from build123d import *

# Parameters (mm, degrees)
SKETCH_1_W      = 22.8
SKETCH_1_H      = 11.8
EXTRUDE_1_DEPTH = 22.6
SKETCH_2_R      = 5.9
EXTRUDE_2_DEPTH = 2.6
SKETCH_3_R      = 2.275
EXTRUDE_3_DEPTH = 2.6
EXTRUDE_4_DEPTH = 2.6
EXTRUDE_5_DEPTH = 2.5
SKETCH_6_W      = 1.6
SKETCH_6_H      = 4
EXTRUDE_6_DEPTH = 1.5
FILLET_1_R      = 0.4


with BuildPart() as part:
    # Эскиз1 → Бобышка-Вытянуть1 (new body)
    with BuildSketch(Plane.XY):
        Rectangle(SKETCH_1_W, SKETCH_1_H)
    extrude(amount=EXTRUDE_1_DEPTH)

    # Эскиз2 → Бобышка-Вытянуть2 (add)
    with BuildSketch(Plane.XY.offset(22.6)):
        with Locations((-5.5, 0)):
            Circle(SKETCH_2_R)
    extrude(amount=EXTRUDE_2_DEPTH)

    # Эскиз3 → Бобышка-Вытянуть3 (add)
    with BuildSketch(Plane.XY.offset(25.2)):
        with Locations((-5.5, 0)):
            Circle(SKETCH_3_R)
    extrude(amount=EXTRUDE_3_DEPTH)

    # Эскиз4 → Бобышка-Вытянуть4 (add)
    with BuildSketch(Plane.XY.offset(22.6)):
        with BuildLine():
            ThreePointArc((-0.419607843, 2.999935921), (-3.4, 0), (-0.419607843, -2.999935921))
            ThreePointArc((-0.419607843, -2.999935921), (0.4, 0), (-0.419607843, 2.999935921))
        make_face()
        with BuildLine():
            ThreePointArc((-0.419607843, 2.999935921), (0.4, 0), (-0.419607843, -2.999935921))
            ThreePointArc((-0.419607843, -2.999935921), (1.714376559, -2.128241472), (2.6, 0))
            ThreePointArc((2.6, 0), (1.714376559, 2.128241472), (-0.419607843, 2.999935921))
        make_face()
    extrude(amount=EXTRUDE_4_DEPTH)

    # Эскиз5 → Бобышка-Вытянуть5 (add)
    with BuildSketch(Plane(origin=(0, 0, 15.9), x_dir=(-1, 0, 0), z_dir=(0, 0, -1))):
        with BuildLine():
            Line((16.2, 5.9), (-16.2, 5.9))
            Line((-16.2, 5.9), (-16.2, 0.65))
            Line((-16.2, 0.65), (-14.659934208, 0.65))
            ThreePointArc((-14.659934208, 0.65), (-12.9, 0), (-14.659934208, -0.65))
            Line((-14.659934208, -0.65), (-16.2, -0.65))
            Line((-16.2, -0.65), (-16.2, -5.9))
            Line((-16.2, -5.9), (16.2, -5.9))
            Line((16.2, -5.9), (16.2, -0.65))
            Line((16.2, -0.65), (14.659934208, -0.65))
            ThreePointArc((14.659934208, -0.65), (12.9, 0), (14.659934208, 0.65))
            Line((14.659934208, 0.65), (16.2, 0.65))
            Line((16.2, 0.65), (16.2, 5.9))
        make_face()
    extrude(amount=-EXTRUDE_5_DEPTH)

    # Эскиз6 → Бобышка-Вытянуть6 (add)
    with BuildSketch(Plane.ZY.offset(11.4)):
        with Locations((5.3, 0)):
            Rectangle(SKETCH_6_W, SKETCH_6_H)
    extrude(amount=EXTRUDE_6_DEPTH)

    # Скругление1
    fillet_1_edges = [part.edges().sort_by_distance(p)[0] for p in [
        (-12.15, -2, 6.1),
        (-12.15, 2, 6.1),
        (-12.15, 2, 4.5),
        (-12.15, -2, 4.5),
        (-12.9, 0, 6.1),
        (-12.9, 2, 5.3),
        (-12.9, 0, 4.5),
        (-12.9, -2, 5.3),
    ]]
    fillet(fillet_1_edges, radius=FILLET_1_R)


solid = part.part
Check sheet for the modelled part. Datum: model origin and axes. Units: mm. A direction names the side the tool comes from. Round coordinates to 2 decimals unless told otherwise and drop trailing zeros. Loops run counter-clockwise (first coordinate to the right, second up) from the corner with the lowest first, then second, coordinate; pieces in that order, holes last. Notation, with made-up numbers: (67, 55) -> (91, 55) arc R15 ccw to (91, 75) -> close; hole circle Ø8 at (15.25, 37). An arc over 180 degrees is marked (long way). Put each result on its own line as item: value. Start each with the question number.
1. Draft check along Z on faces 1 (the face through (0, -5.9, 11)), 2 (the face through (-12, 0, 6.1)), 3 (the face through (-6, 0, 27.8)). Enter one of: +Z half, -Z half, draft (parallel to the pull), parting line (faces both ways), or undercut.
2. Section check B-B (z = 17.5). Enter the section's corners in (x, y).
3. Section check A-A (x = -13.9). Enter the section's corners in (y, z).
4. Scan lines: probe 1 along Y at (x, z) = (-13.9, 16.4); probe 2 along Z at (x, y) = (-12, 1); probe 3 along Z at (x, y) = (6, -5.25). Record each from-to range of solid material in increasing order.
5. Gauge pin test, flat ends, axial feed: pin 1 (0.6 mm diameter, centred on x = -12, z = 5.5, fed in from +Y); pin 2 (6.5 mm diameter, centred on x = -9.5, y = 2, fed in from +Z); pin 3 (5 mm diameter, centred on y = -4, z = 6.5, fed in from -X); pin 4 (0.5 mm diameter, centred on x = -12, y = 0.5, fed in from -Z). Record the tip position at first contact, or that the pin passes through.
6. Access from +Z, -Z, +X, -X, +Y, -Y to the whole of each face (thin tool, end or side, straight path). Record for faces 4 (the face through (-11.396, 0.215, 23.882)), 5 (the face through (15, 0.65, 17)), 6 (the face through (-10.2, 4.5, 22.6)), 7 (the face through (-15, -0.65, 17)).
7. Section check C-C (y = 3.75). Enter the section's corners in (x, z), plus the area to 3 significant figures.
8. Section check D-D (x = -4.5). Enter the section's corners in (y, z).
Findings:
1. face 1: draft
1. face 2: undercut
1. face 3: +Z half
2. outline: (-16.2, -5.9) -> (16.2, -5.9) -> (16.2, -0.65) -> (14.66, -0.65) arc R1 cw (long way) to (14.66, 0.65) -> (16.2, 0.65) -> (16.2, 5.9) -> (-16.2, 5.9) -> (-16.2, 0.65) -> (-14.66, 0.65) arc R1 cw (long way) to (-14.66, -0.65) -> (-16.2, -0.65) -> close
3. outline: (-5.9, 15.9) -> (-1, 15.9) -> (-1, 18.4) -> (-5.9, 18.4) -> close; (1, 15.9) -> (5.9, 15.9) -> (5.9, 18.4) -> (1, 18.4) -> close
4. probe 1: y = -5.9 to -1, 1 to 5.9
4. probe 2: z = 4.5 to 6.1, 15.9 to 18.4
4. probe 3: z = 0 to 22.6
5. pin 1: stops at y = 2
5. pin 2: stops at z = 27.8
5. pin 3: stops at x = -12.9
5. pin 4: stops at z = 4.5
6. face 4: +Z
6. face 5: +Z, -Z, +X
6. face 6: +Z, -X, +Y
6. face 7: +Z, -Z, -X
7. outline: (-16.2, 15.9) -> (-11.4, 15.9) -> (-11.4, 0) -> (11.4, 0) -> (11.4, 15.9) -> (16.2, 15.9) -> (16.2, 18.4) -> (11.4, 18.4) -> (11.4, 22.6) -> (-0.95, 22.6) -> (-0.95, 25.2) -> (-10.05, 25.2) -> (-10.05, 22.6) -> (-11.4, 22.6) -> (-11.4, 18.4) -> (-16.2, 18.4) -> close
7. area: 563 mm^2
8. outline: (-5.9, 0) -> (5.9, 0) -> (5.9, 22.6) -> (5.81, 22.6) -> (5.81, 25.2) -> (2.04, 25.2) -> (2.04, 27.8) -> (-2.04, 27.8) -> (-2.04, 25.2) -> (-5.81, 25.2) -> (-5.81, 22.6) -> (-5.9, 22.6) -> close
